Check sheet for the modelled part. Datum: model origin and axes. Units: mm. Round coordinates to 2 decimals unless told otherwise and drop trailing zeros. Loops run counter-clockwise (first coordinate to the right, second up) from the corner with the lowest first, then second, coordinate; pieces in that order, holes last. Notation, with made-up numbers: (28.25, 74) - (80.25, 74) arc R15 cw to (80.25, 93) - close; hole circle Ø8 at (68, 54). An arc over 180 degrees is marked (long way). Put each result on its own line as item: value. Start each with the question number.
Autodesk Inventor part; units mm, degrees
ref_plane "YZ Plane" through (0, 0, 0) normal (1, 0, 0) x (0, 1, 0)
ref_plane "XZ Plane" through (0, 0, 0) normal (0, 1, 0) x (-1, 0, 0)
ref_plane "XY Plane" through (0, 0, 0) normal (0, 0, 1) x (1, 0, 0)
sketch "Sketch1" plane through (0, 0, 0) normal (0, 1, 0) x (-1, 0, 0)
  line L0 (135, 97.5) -> (-135, 97.5)
  line L1 (-135, 97.5) -> (-135, -97.5)
  line L2 (-135, -97.5) -> (135, -97.5)
  line L3 (135, -97.5) -> (135, 97.5)
  line L4 (135, 97.5) -> (-135, -97.5) construction
  line L5 (-135, 97.5) -> (135, -97.5) construction
  line L6 (135, 97.5) -> (-5, 97.5)
  line L7 (-5, 97.5) -> (-5, 109.5)
  line L8 (-5, 109.5) -> (135, 109.5)
  line L9 (135, 109.5) -> (135, 97.5)
  point P0 (0, 0)
  dimension "d0" = 270
  dimension "d1" = 195
  dimension "d2" = 140
  dimension "d3" = 12
  dimension "d4" = 0
  dimension "d5" = 0
extrude "Extrusion1" add sketch "Sketch1" along normal blind 2.5
sketch "Sketch2" plane through (0, 2.5, 0) normal (0, 1, 0) x (1, 0, 0)
  line L0 (26.75, -17.5) -> (119.25, -17.5) construction
  line L1 (119.25, -17.5) -> (119.25, -87.5) construction
  line L2 (119.25, -87.5) -> (26.75, -87.5) construction
  line L3 (26.75, -87.5) -> (26.75, -17.5) construction
  line L4 (26.75, -17.5) -> (119.25, -87.5) construction
  line L5 (119.25, -17.5) -> (26.75, -87.5) construction
  line L6 (5, -97.5) -> (135, -97.5) construction
  line L7 (135, -97.5) -> (135, 97.5)
  point P0 (0, 0)
  point P1 (73, -52.5)
  dimension "d8" = 92.5
  dimension "d9" = 70
  dimension "d10" = 45
  dimension "d11" = 62
hole "LRS-35-5" at (26.75, 2.5, 17.5) at (119.25, 2.5, 87.5) direction (0, -1, 0) diameter 2.459 end through all
sketch "HB12-1.7AG" plane through (0, 2.5, 0) normal (0, 1, 0) x (1, 0, 0)
  line L0 (-115, -103.5) -> (-10.2, -103.5) construction
  line L1 (-10.2, -103.5) -> (-10.2, -17.8) construction
  line L2 (-10.2, -17.8) -> (-115, -17.8) construction
  line L3 (-115, -17.8) -> (-115, -103.5) construction
  line L4 (-115, -103.5) -> (-10.2, -17.8) construction
  line L5 (-10.2, -103.5) -> (-115, -17.8) construction
  line L6 (-135, 97.5) -> (-135, -109.5) construction
  line L7 (-135, -109.5) -> (5, -109.5) construction
  point P0 (0, 0)
  point P1 (-62.6, -60.65)
  dimension "d19" = 104.8
  dimension "d20" = 85.7
  dimension "d23" = 6
  dimension "d24" = 20
hole "BEl PSU" at (-115, 2.5, 17.8) at (-10.2, 2.5, 17.8) at (-10.2, 2.5, 103.5) at (-115, 2.5, 103.5) at (-115, 2.5, 17.8) at (-10.2, 2.5, 17.8) at (-10.2, 2.5, 103.5) at (-115, 2.5, 103.5) direction (0, -1, 0) diameter 2.459 end through all
sketch "Mounting Holes" plane through (0, 2.5, 0) normal (0, 1, 0) x (1, 0, 0)
  line L0 (-127, -88.9) -> (127, -88.9) construction
  line L1 (127, -88.9) -> (127, 88.9) construction
  line L2 (127, 88.9) -> (-127, 88.9) construction
  line L3 (-127, 88.9) -> (-127, -88.9) construction
  line L4 (-127, -88.9) -> (127, 88.9) construction
  line L5 (127, -88.9) -> (-127, 88.9) construction
  point P0 (0, 0)
  dimension "d32" = 254
  dimension "d33" = 177.8
hole "Hole3" at (-127, 2.5, -88.9) at (127, 2.5, -88.9) at (127, 2.5, 88.9) at (-127, 2.5, 88.9) direction (0, -1, 0) diameter 4.5 end through all
sketch "WR-LEN" plane through (0, 2.5, 0) normal (0, 1, 0) x (1, 0, 0)
  line L0 (32.5, 80.5) -> (-57.5, 80.5) construction
  line L1 (-57.5, 80.5) -> (-57.5, 10.5) construction
  line L2 (-57.5, 10.5) -> (32.5, 10.5) construction
  line L3 (32.5, 10.5) -> (32.5, 80.5) construction
  line L4 (32.5, 80.5) -> (-57.5, 10.5) construction
  line L5 (-57.5, 80.5) -> (32.5, 10.5) construction
  line L6 (-135, 97.5) -> (-135, -109.5)
  line L7 (135, 97.5) -> (-135, 97.5)
  point P0 (0, 0)
  point P1 (-12.5, 45.5)
  dimension "d41" = 90
  dimension "d42" = 70
  dimension "d44" = 52
  dimension "d52" = 77.5
hole "WR-LEN-Hole" at (-57.5, 2.5, -80.5) at (32.5, 2.5, -80.5) at (32.5, 2.5, -10.5) at (-57.5, 2.5, -10.5) direction (0, -1, 0) diameter 2.459 end through all
sketch "GND" plane through (0, 2.5, 0) normal (0, 1, 0) x (1, 0, 0)
  line L0 (135, -97.5) -> (135, 97.5)
  line L1 (135, 97.5) -> (-135, 97.5)
  point P0 (0, 0)
  point P1 (115, 0)
  dimension "d53" = 20
  dimension "d54" = 97.5
hole "GND-Hole" at (115, 2.5, 0) direction (0, -1, 0) diameter 3.242 end through all
properties part number "Plate-0"
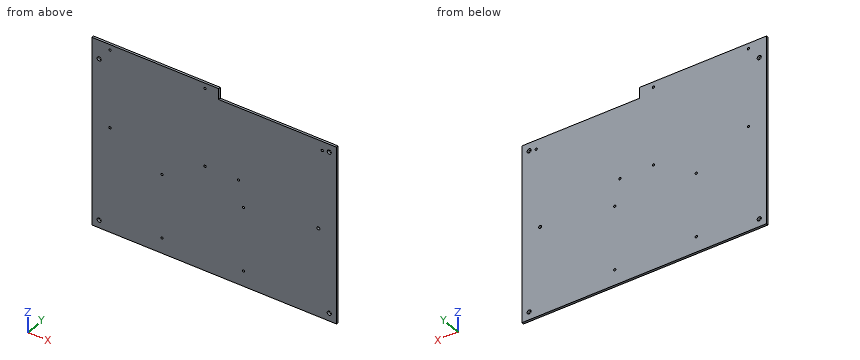
Q1. Cross-section at B-B on x = 78. Enter the section's corners in (y, z).
Q2. Depth check by flat-ended pin: pin 1 Ø2.5 at (x, z) = (127, 88.9) entering from -Y; pin 2 Ø3 at (x, z) = (-115, 103.5) entering from +Y; pin 3 Ø1.2 at (x, y) = (88.5, 1.5) entering from +Z. Enter the tip coordinate at first touch or a pass-through.
Q3. Cross-section at A-A on y = 1.85. State how many separate pieces and enclosed holes the cut face has, and give its area (3 significant figures).
Q4. Material ranges on line 1 (X direction, y = 1.85, z = 88.9); line 2 (X direction, y = 1.8, z = -80.5); line 3 (Z direction, x = -127, y = 1.4), recorded low to high. Write a range as from..to.
Answer list:
1. outline: (0, -97.5) - (2.5, -97.5) - (2.5, 97.5) - (0, 97.5) - close
2. pin 1: passes through
2. pin 2: stops at y = 2.5
2. pin 3: stops at z = 97.5
3. separate pieces: 1
3. enclosed holes: 15
3. area: 54,200 mm2
4. line 1: x = -135..-129.25, -124.75..124.75, 129.25..135
4. line 2: x = -135..-58.73, -56.27..31.27, 33.73..135
4. line 3: z = -97.5..-91.15, -86.65..86.65, 91.15..109.5
